from build123d import *

# Parameters (mm, degrees)
SKETCH4_W           = 76.2
SKETCH4_H           = 3.175
BOSS_EXTRUDE4_DEPTH = 50.8
SKETCH5_W           = 7.35
SKETCH5_H           = 49.462905427
BOSS_EXTRUDE5_DEPTH = 8.525
SKETCH6_R           = 4.2625
BOSS_EXTRUDE6_DEPTH = 6.85
FILLET1_R           = 1
FILLET2_R           = 3.54


with BuildPart() as part:
    # Sketch4 → Boss-Extrude4 (new body)
    with BuildSketch(Plane.XY):
        with Locations((0, 1.5875)):
            Rectangle(SKETCH4_W, SKETCH4_H)
    extrude(amount=BOSS_EXTRUDE4_DEPTH)

    # Sketch5 → Boss-Extrude5 (add)
    with BuildSketch(Plane(origin=(0, 0, 0), x_dir=(1, 0, 0), z_dir=(0, 0.069756474, 0.99756405))):
        Polygon((-3.712235216, 0), (-6.887235216, 0), (-6.887235216, -139.7), (-3.712235216, -139.7), (-3.712235216, -81.218439027), (3.637764784, -81.218439027), (3.637764784, -139.7), (6.812764784, -139.7), (6.812764784, 0), (3.637764784, 0), (3.637764784, -28.5805336), (-3.712235216, -28.5805336), align=None)
        with Locations((-0.037235216, -54.899486314)):
            Rectangle(SKETCH5_W, SKETCH5_H, mode=Mode.SUBTRACT)
    extrude(amount=BOSS_EXTRUDE5_DEPTH)

    # Sketch6 → Boss-Extrude6 (add)
    with BuildSketch(Plane(origin=(-3.712235216, 0, 0), x_dir=(0, 0, -1), z_dir=(1, 0, 0))):
        with Locations((-13.699759177, -134.810244088)):
            Circle(SKETCH6_R)
    extrude(amount=BOSS_EXTRUDE6_DEPTH)

    # Fillet1
    fillet1_edges = [part.edges().sort_by_distance(p)[0] for p in [
        (5.225264784, 0, 8.545817181),
        (-5.299735216, 0, 8.545817181),
        (3.637764784, 0, 4.272908591),
        (-6.887235216, 0, 4.272908591),
        (-3.712235216, -28.213575887, 6.245794006),
        (-3.712235216, -29.797208817, 6.356532408),
        (3.637764784, -28.213575887, 6.245794006),
        (-3.712235216, -80.723258022, 9.917628674),
        (3.637764784, -79.139625092, 9.806890272),
        (3.637764784, -29.797208817, 6.356532408),
        (-3.712235216, -79.139625092, 9.806890272),
        (-3.712235216, 0, 4.272908591),
        (3.637764784, -80.723258022, 9.917628674),
        (6.812764784, 0, 4.272908591),
    ]]
    fillet(fillet1_edges, radius=FILLET1_R)

    # Fillet2
    fillet2_edges = [part.edges().sort_by_distance(p)[0] for p in [
        (-5.299735216, -138.765023883, 18.249212911),
        (5.225264784, -138.765023883, 18.249212911),
        (-5.299735216, -139.359697821, 9.744979382),
        (5.225264784, -139.359697821, 9.744979382),
    ]]
    fillet(fillet2_edges, radius=FILLET2_R)


solid = part.part
The listing builds one solid part. Answer for the finished solid, in the listing's coordinates (mm). A direction names the side the tool comes from. Give positions to 0.01 mm unless a question says otherwise; leave off trailing zeros. Loops run counter-clockwise (first coordinate to the right, second up) from the corner with the lowest first, then second, coordinate; pieces in that order, holes last.
Item 1: Determine the mould class of faces 1 (the flat face through (-1, 3.175, 25)), 2 (the flat face through (-3.712, -14, 5)), 3 (the flat face through (-38.1, 2, 25)), 4 (the cylindrical face through (5.25, -138.28, 10.74)) for opening direction Y: +Y half, -Y half, draft (parallel to the pull), parting line (faces both ways), or undercut.
Derived:
face 1: +Y half
face 2: undercut
face 3: draft
face 4: -Y half
Item 2: Each of these flat-tipped pins is pushed along its axis until it touches: pin 1 Ø2 at (y, z) = (-138, 16.5) entering from +X; pin 2 Ø15 at (x, z) = (-17, 24) entering from -Y; pin 3 Ø9 at (y, z) = (-66, 12) entering from -X. Where does it stop, or does it pass through?
Derived:
pin 1: stops at x = 6.81
pin 2: stops at y = 0
pin 3: stops at x = -6.89
Item 3: A cutting plane is placed at D-D (z = 36.5). Give the vertices of the cut face in (x, y) (3 decimals), then the cut area to 3 significant figures.
Derived:
outline: (-38.1, 0) - (38.1, 0) - (38.1, 3.175) - (-38.1, 3.175) - close
area: 242 mm2
Item 4: A cutting plane is placed at C-C (x = 23). Give the vertices of the cut face in (y, z) (3 decimals), then the cut area to 3 significant figures.
Derived:
outline: (0, 0) - (3.175, 0) - (3.175, 50.8) - (0, 50.8) - close
area: 161 mm2
Item 5: Find the intervals of material crossed by line 1 along X through (y, z) = (-101, 11.5); line 2 along Y through (x, z) = (3.5, 24) (3 decimals); line 3 along Z through (x, y) = (-6.5, -39), in increasing order.
Derived:
line 1: x = -6.89 to -3.71, 3.64 to 6.81
line 2: y = 0 to 3.175
line 3: z = 2.73 to 11.27
Item 6: A tool of negligible diameter and unlimited length cuts with its end or side. For faces 5 (the flat face through (-0.075, -79.144, 9.747)), 6 (the flat face through (-6.887, -69, 9)), 7 (the flat face through (-3.712, -55, 8)), 8 (the flat face through (6.813, -71, 9)), from which of +Z, -Z, +X, -X, +Y, -Y can it reach the whole face along a straight path? Write none if from no direction.
Derived:
face 5: -Z
face 6: +Z, -Z, -X, -Y
face 7: +Z, -Z
face 8: +Z, -Z, +X, -Y
Item 7: A cutting plane is placed at A-A (x = -1). Give the vertices of the cut face in (y, z) (1 decimal).
Derived:
outline: circle Ø8.5 at (-134.8, 13.7); (-81, 5.7) - (-79.4, 5.6) - (-78.8, 14.1) - (-80.4, 14.2) - close; (-30.1, 2.1) - (-28.5, 2) - (-27.9, 10.5) - (-29.5, 10.6) - close; (0, 0) - (3.2, 0) - (3.2, 50.8) - (0, 50.8) - close
Item 8: A cutting plane is placed at B-B (y = -61.5). Give the vertices of the cut face in (x, z).
Derived:
outline: (-6.89, 4.3) - (-3.71, 4.3) - (-3.71, 12.85) - (-6.89, 12.85) - close; (3.64, 4.3) - (6.81, 4.3) - (6.81, 12.85) - (3.64, 12.85) - close
